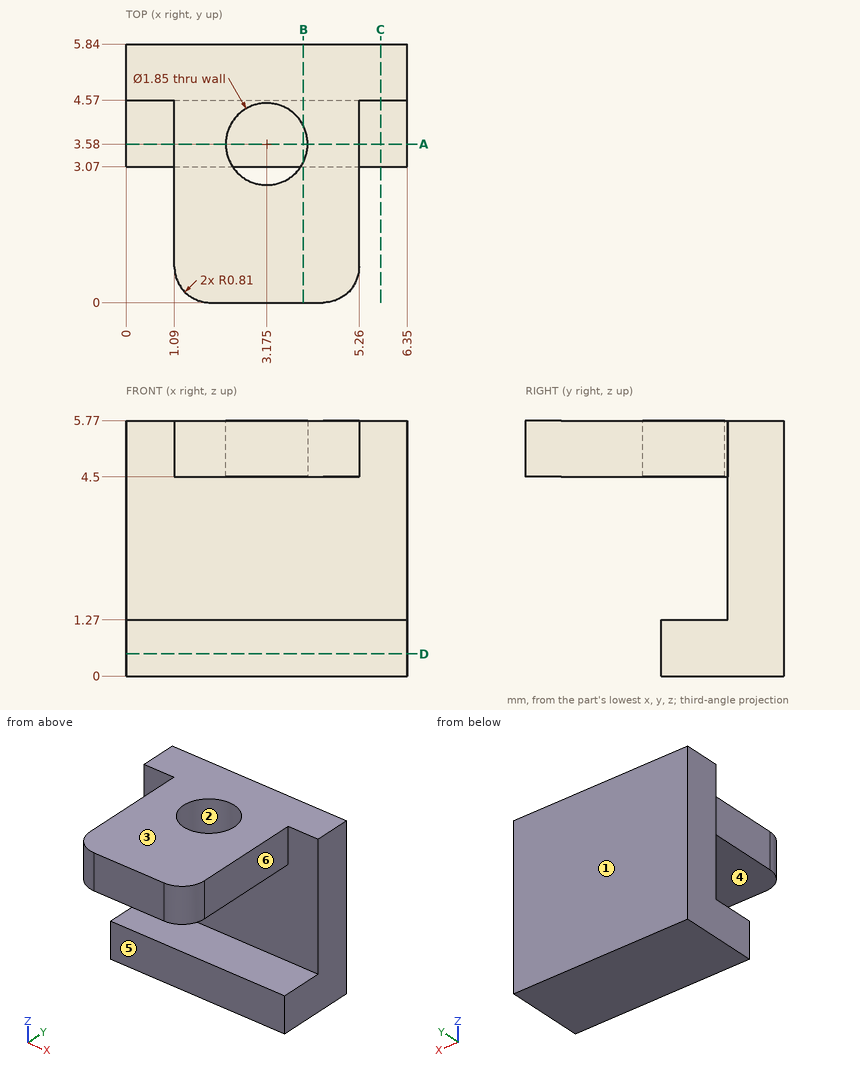
Design review of the part shown in the three views and the two pictorial views. Dimensions are in mm from the part's minimum x, y and z. A direction names the side the tool comes from. Round coordinates to 2 decimals unless told otherwise and drop trailing zeros. Order: outer loops, then holes, each group sorted by start corner. A loop starts at its lowest first (then second) coordinate and runs counter-clockwise, first axis right, second up. Notation, with made-up numbers: (0, 29) - (59, 29) arc R35 ccw to (59, 68) - close; hole circle Ø8 at (56.5, 60). An arc over 180 degrees is marked (long way). Answer in a Markdown table with one row per item.
(1) Take a section at C-C on x = 5.75. Write out the cut boundary in (y, z), plus the area to 3 significant figures.
Result set:
| item | result |
|---|---|
| outline | (3.07, 0) - (5.84, 0) - (5.84, 5.77) - (4.57, 5.77) - (4.57, 1.27) - (3.07, 1.27) - close |
| area | 9.23 mm2 |
(2) Machinability: for the marked faces 4, 5 and 6, which of the approach directions +Z, -Z, +X, -X, +Y, -Y give a long, thin tool a straight path to every point of the face, cutting with its end or side? Answer none if there is none.
Result set:
| item | result |
|---|---|
| face 4 | +X, -X, -Y |
| face 5 | -Z, +X, -X, -Y |
| face 6 | +Z, +X, -Y |
(3) Take a section at A-A on y = 3.58. Write out the cut boundary in (x, z), plus the area to 3 significant figures.
Result set:
| item | result |
|---|---|
| outline | (0, 0) - (6.35, 0) - (6.35, 1.27) - (0, 1.27) - close; (1.09, 4.5) - (2.25, 4.5) - (2.25, 5.77) - (1.09, 5.77) - close; (4.1, 4.5) - (5.26, 4.5) - (5.26, 5.77) - (4.1, 5.77) - close |
| area | 11.0 mm2 |
(4) Take a section at B-B on x = 4. Write out the cut boundary in (y, z).
Result set:
| item | result |
|---|---|
| outline | (0, 4.5) - (3.16, 4.5) - (3.16, 5.77) - (0, 5.77) - close; (3.07, 0) - (5.84, 0) - (5.84, 5.77) - (4, 5.77) - (4, 4.5) - (4.57, 4.5) - (4.57, 1.27) - (3.07, 1.27) - close |
(5) Clearance check with flat-ended pins moving along their axes: P1, Ø1, axis at x = 2, z = 0.5, coming from the -Y side; P2, Ø1.4, axis at y = 3.5, z = 5, coming from the -X side; P3, Ø1.4, axis at y = 3.5, z = 5.5, coming from the +X side. State where each tip first meets the part, or that it passes through.
Result set:
| item | result |
|---|---|
| P1 | stops at y = 3.07 |
| P2 | stops at x = 1.09 |
| P3 | stops at x = 5.26 |
(6) Mouldability with a two-part tool opening along Y and no side actions: class the marked faces 1, 2 and 3 as released by +Y, released by -Y, zero draft, split by the parting line, or undercut.
Result set:
| item | result |
|---|---|
| face 1 | released by +Y |
| face 2 | undercut |
| face 3 | zero draft |
(7) For line 1 (Y direction, x = 2, z = 2.7); line 2 (Y direction, x = 5, z = 0.7); line 3 (Y direction, x = 4, z = 5), list the stretches that pass through material, from the lowest coordinate up. Write a range as from..to.
Result set:
| item | result |
|---|---|
| line 1 | y = 4.57..5.84 |
| line 2 | y = 3.07..5.84 |
| line 3 | y = 0..3.16, 4..5.84 |
(8) Take a section at D-D on z = 0.5. Write out the cut boundary in (x, y).
Result set:
| item | result |
|---|---|
| outline | (0, 3.07) - (6.35, 3.07) - (6.35, 5.84) - (0, 5.84) - close |
